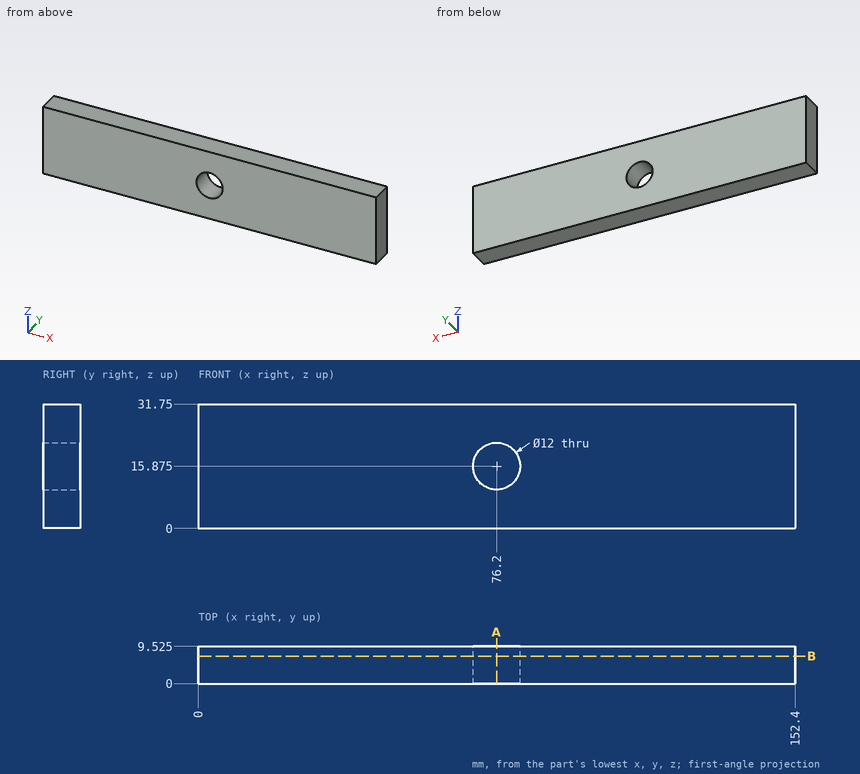
The drawing under review shows one solid part. Ordinate dimensions are in mm from its lowest x, y, z. Give positions to 0.01 mm unless a question says otherwise; leave off trailing zeros. Order: outer loops, then holes, each group sorted by start corner. A loop starts at its lowest first (then second) coordinate and runs counter-clockwise, first axis right, second up. Notation, with made-up numbers: M 70.5,13.5 L 79.5,13.5 A21 ccw 79.5,36.5 Z; hole C -16.5,72 d3. An arc over 180 degrees is marked long. Answer in a Markdown table with one row per item. Add a question column.
1. To check wall thickness, follow line 1 along Z through (x, y) = (76.2, 4.5) (3 decimals); line 2 along X through (y, z) = (6.75, 14); line 3 along X through (y, z) = (8.5, 20.5). State the ranges of each line that lie inside material, in increasing order.
2. Add section B-B on y = 7. State the section outline as (x, z) points (3 decimals).
3. Add section A-A on x = 76.2. State the section outline as (y, z) points (3 decimals), plus the area to 3 significant figures.
The answers:
| question | item | result |
|---|---|---|
| 1 | line 1 | 0 to 9.875, 21.875 to 31.75 |
| 1 | line 2 | 0 to 70.5, 81.9 to 152.4 |
| 1 | line 3 | 0 to 72.38, 80.02 to 152.4 |
| 2 | outline | M 0,0 L 152.4,0 L 152.4,31.75 L 0,31.75 Z; hole C 76.2,15.875 d12 |
| 3 | outline | M 0,0 L 9.525,0 L 9.525,9.875 L 0,9.875 Z; M 0,21.875 L 9.525,21.875 L 9.525,31.75 L 0,31.75 Z |
| 3 | area | 188 mm2 |
